```python
from build123d import *

# Parameters (mm, degrees)
F0_R     = 5.55625
F1_DEPTH = 25.4
F2_W     = 25.4
F2_H     = 57.15
F3_DEPTH = 38.1
F4_R     = 6.35
F5_R     = 7.9375
F6_DEPTH = 25.4


with BuildPart() as f1:
    # F0 (on Front) → F1 (new body)
    with BuildSketch(Plane.XZ):
        with BuildLine():
            ThreePointArc((0, 6.35), (1.859872, 1.859872), (6.35, 0))
            Line((6.35, 0), (54.359485, 0))
            ThreePointArc((54.359485, 0), (58.707315, 1.721947), (60.697119, 5.953898))
            Line((60.697119, 5.953898), (63.078369, 44.053898))
            ThreePointArc((63.078369, 44.053898), (61.368788, 48.79783), (56.740735, 50.8))
            Line((56.740735, 50.8), (6.35, 50.8))
            ThreePointArc((6.35, 50.8), (1.859872, 48.940128), (0, 44.45))
            Line((0, 44.45), (0, 6.35))
        make_face()
        with Locations((12.7, 25.4)):
            Circle(F0_R, mode=Mode.SUBTRACT)
        with Locations((50.8, 25.4)):
            Circle(F0_R, mode=Mode.SUBTRACT)
    extrude(amount=F1_DEPTH)

    # F2 (on face) → F3 (join)
    with BuildSketch(Plane.XY.offset(50.8)):
        with Locations((31.75, -28.575)):
            Rectangle(F2_W, F2_H)
    extrude(amount=F3_DEPTH)

    # F4
    f4_edges = [f1.edges().sort_by_distance(p)[0] for p in [
        (31.75, -57.15, 88.9),
        (31.75, -57.15, 50.8),
        (31.75, 0, 88.9),
    ]]
    fillet(f4_edges, radius=F4_R)

    # F5 (on face) → F6 (cut)
    with BuildSketch(Plane(origin=(19.05, 0, 0), x_dir=(0, -1, 0), z_dir=(-1, 0, 0))):
        with Locations((44.45, 69.85)):
            Circle(F5_R)
    extrude(amount=-F6_DEPTH, mode=Mode.SUBTRACT)


solid = f1.part
```
Design review of the part built by this model. Coordinates are the model's own, in mm. A direction names the side the tool comes from. Coordinates: 2 decimals unless noted, no trailing zeros. Order: outer loops, then holes, each group sorted by start corner. A loop starts at its lowest first (then second) coordinate and runs counter-clockwise, first axis right, second up. Notation, with made-up numbers: (24, -16.75) -> (37, -16.75) arc R23 ccw to (37, -8.75) -> close; hole circle Ø10 at (52, -16). An arc over 180 degrees is marked (long way). One line per item, written item: value. Start each with the question number.
Q1. Insertion check: pin 1 Ø11.5 at (y, z) = (-18.5, 70) entering from +X; pin 2 Ø7.5 at (x, y) = (30.5, -33) entering from -Z; pin 3 Ø18 at (x, z) = (12.7, 25.4) entering from -Y. Each pin has a flat end and moves straight along its axis. Give the tip position at first contact, or say it passes through.
Q2. For probe 1 along X at (y, z) = (-15, 25); probe 2 along Z at (x, y) = (50.8, -9.5); probe 3 along Z at (x, y) = (38.25, -44.45), list the stretches that pass through material, from the lowest coordinate up.
Q3. Take a section at C-C, the plane y = -14. State the section outline as (x, z) points.
Q4. Tool access review of faces 1 (the flat face through (61.87, -12.52, 24.74)), 2 (the flat face through (32, -38, 50.8)), 3 (the flat face through (13, -13, 50.8)): name each direction out of +Z, -Z, +X, -X, +Y, -Y from which nothing blocks a thin tool from reaching the whole face with its end or side.
Q5. Mouldability with a two-part tool opening along Z and no side actions: class faces 4 (the flat face through (0, -13, 26)), 5 (the cylindrical face through (31.93, -55.34, 52.71)), 6 (the flat face through (51, -13, 50.8)), 7 (the cylindrical face through (31.57, -38.15, 65.02)) as pulls with the +Z half, pulls with the -Z half, needs draft (parallel to the pull), parting line crosses it, or undercut.
Q6. Take a section at A-A, the plane y = -44.45. State the section outline as (x, z) points, then the cut area to 3 significant figures.
Q7. Take a section at D-D, the plane z = 69.85. State the section outline as (x, y) points.
Q8. Take a section at B-B, the plane z = 25.4. State the section outline as (x, y) points, then the cut area to 3 significant figures.
Values follow:
1. pin 1: stops at x = 44.45
1. pin 2: stops at z = 50.8
1. pin 3: stops at y = -25.4
2. probe 1: x = 0 to 7.16, 18.24 to 45.26, 56.34 to 61.89
2. probe 2: z = 0 to 19.84, 30.96 to 50.8
2. probe 3: z = 50.8 to 61.91, 77.79 to 88.9
3. outline: (0, 6.35) arc R6.35 ccw to (6.35, 0) -> (54.36, 0) arc R6.35 ccw to (60.7, 5.95) -> (63.08, 44.05) arc R6.35 ccw to (56.74, 50.8) -> (44.45, 50.8) -> (44.45, 88.9) -> (19.05, 88.9) -> (19.05, 50.8) -> (6.35, 50.8) arc R6.35 ccw to (0, 44.45) -> close; hole circle Ø11.11 at (12.7, 25.4); hole circle Ø11.11 at (50.8, 25.4)
4. face 1: -Z, +X, +Y, -Y
4. face 2: -Z, +X, -X, -Y
4. face 3: +Z, -X, +Y, -Y
5. face 4: needs draft
5. face 5: pulls with the -Z half
5. face 6: pulls with the +Z half
5. face 7: undercut
6. outline: (19.05, 50.8) -> (44.45, 50.8) -> (44.45, 61.91) -> (19.05, 61.91) -> close; (19.05, 77.79) -> (44.45, 77.79) -> (44.45, 88.9) -> (19.05, 88.9) -> close
6. area: 565 mm2
7. outline: (19.05, -57.15) -> (44.45, -57.15) -> (44.45, -52.39) -> (19.05, -52.39) -> close; (19.05, -36.51) -> (44.45, -36.51) -> (44.45, 0) -> (19.05, 0) -> close
8. outline: (0, -25.4) -> (7.14, -25.4) -> (7.14, 0) -> (0, 0) -> close; (18.26, -25.4) -> (45.24, -25.4) -> (45.24, 0) -> (18.26, 0) -> close; (56.36, -25.4) -> (61.91, -25.4) -> (61.91, 0) -> (56.36, 0) -> close
8. area: 1,010 mm2
